Input: part model. Units: mm. Frame: model coordinates. A direction names the side the tool comes from. Round coordinates to 2 decimals unless told otherwise and drop trailing zeros. Loops run counter-clockwise (first coordinate to the right, second up) from the corner with the lowest first, then second, coordinate; pieces in that order, holes last. Notation, with made-up numbers: (-2, 27.5) -> (24, 27.5) arc R28 cw to (24, 65.5) -> close; hole circle Ø10 at (-1, -37.5). An arc over 180 degrees is marked (long way). Answer in a Markdown table with one row per item. Add a question column.
Q1. Pin query (flat end, axial travel): pin 1 (1.8 mm diameter, centred on x = 4.5, y = 4.5, fed in from -Z); pin 2 (2.5 mm diameter, centred on x = 2, z = -58, fed in from -Y); pin 3 (9 mm diameter, centred on y = 15.25, z = -4, fed in from +X). Return the tip coordinate at first contact, or that it passes through.
Q2. Section C-C, the plane y = 21.25. Output: boundary loops of the cut face in (x, z).
Q3. Ray query, L1, parallel to Z at x = 2.4, y = 15.25; L2, parallel to Z at x = 2.3, y = 18.25; L3, parallel to Y at x = 3.8, z = -52. Return the intervals inside material, ascending. Write a range as from..to.
Q4. Reachability of faces 5 (the face through (3, 6.25, 1)), 6 (the face through (3, 6.25, -57)), 7 (the face through (3, 14, -59)), 8 (the face through (3, 22.25, 1)), 9 (the face through (3, 21, -6.25)) from +Z, -Z, +X, -X, +Y, -Y: full face, straight path, thin tool, end or side. Return the list, or none.
Q5. Section D-D, the plane z = -4. Output: boundary loops of the cut face in (x, y).
Q6. Section A-A, the plane y = 15.25. Output: boundary loops of the cut face in (x, z), and give its area (3 significant figures).
Q7. Section B-B, the plane x = 2.8. Output: boundary loops of the cut face in (y, z).
Q8. Mould query, pull axis Z, two halves, no side actions, for faces 1 (the face through (2.958, 10.254, -3.813)), 2 (the face through (3, 3, -56)), 3 (the face through (3, 3, 0)), 4 (the face through (3, 21, -1.75)). Classes: pulls with the +Z half, pulls with the -Z half, needs draft (parallel to the pull), parting line crosses it, or undercut.
```python
from build123d import *

# Parameters (mm, degrees)
SKETCH1_W           = 6
SKETCH1_H           = 56
BOSS_EXTRUDE1_DEPTH = 22.25
SKETCH6_W           = 6
SKETCH6_H           = 16
BOSS_EXTRUDE3_DEPTH = 3
CUT_EXTRUDE1_DEPTH  = 6


with BuildPart() as part:
    # Sketch1 → Boss-Extrude1 (new body)
    with BuildSketch(Plane(origin=(0, 0, 0), x_dir=(1, 0, 0), z_dir=(0, 1, 0))):
        with Locations((3, 28)):
            Rectangle(SKETCH1_W, SKETCH1_H)
    extrude(amount=BOSS_EXTRUDE1_DEPTH)

    # Sketch6 → Boss-Extrude3 (add)
    with BuildSketch(Plane(origin=(0, 0, -56), x_dir=(-1, 0, 0), z_dir=(0, 0, -1))):
        with Locations((-3, 14.25)):
            Rectangle(SKETCH6_W, SKETCH6_H)
    boss_extrude3 = extrude(amount=BOSS_EXTRUDE3_DEPTH)

    # Mirror3: Boss-Extrude3 across plane
    add(boss_extrude3.mirror(Plane(origin=(0, 0, -28), x_dir=(1, 0, 0), z_dir=(0, 0, -1))))

    # Sketch7 → Cut-Extrude1 (cut)
    with BuildSketch(Plane.ZY):
        with BuildLine():
            Line((-54.25, 19.715142775), (-54.25, 24.715142775))
            Line((-54.25, 24.715142775), (-49.75, 24.715142775))
            Line((-49.75, 24.715142775), (-49.75, 19.715142775))
            ThreePointArc((-49.75, 19.715142775), (-52, 10.25), (-54.25, 19.715142775))
        make_face()
        with BuildLine():
            Line((-6.25, 19.715142775), (-6.25, 24.715142775))
            Line((-6.25, 24.715142775), (-1.75, 24.715142775))
            Line((-1.75, 24.715142775), (-1.75, 19.715142775))
            ThreePointArc((-1.75, 19.715142775), (-4, 10.25), (-6.25, 19.715142775))
        make_face()
    extrude(amount=-CUT_EXTRUDE1_DEPTH, mode=Mode.SUBTRACT)


solid = part.part
```
Answer block:
| question | item | result |
|---|---|---|
| 1 | pin 1 | z = -56 |
| 1 | pin 2 | y = 6.25 |
| 1 | pin 3 | through |
| 2 | outline | (0, -59) -> (6, -59) -> (6, -54.25) -> (0, -54.25) -> close; (0, -49.75) -> (6, -49.75) -> (6, -6.25) -> (0, -6.25) -> close; (0, -1.75) -> (6, -1.75) -> (6, 3) -> (0, 3) -> close |
| 3 | L1 | -59..-57, -47..-9, 1..3 |
| 3 | L2 | -59..-56, -48..-8, 0..3 |
| 3 | L3 | 0..10.25 |
| 4 | face 5 | +Z, +X, -X, -Y |
| 4 | face 6 | -Z, +X, -X, -Y |
| 4 | face 7 | -Z, +X, -X, +Y, -Y |
| 4 | face 8 | +Z, -Z, +X, -X, +Y |
| 4 | face 9 | +X, -X, +Y |
| 5 | outline | (0, 0) -> (6, 0) -> (6, 10.25) -> (0, 10.25) -> close |
| 6 | outline | (0, -59) -> (6, -59) -> (6, -57) -> (0, -57) -> close; (0, -47) -> (6, -47) -> (6, -9) -> (0, -9) -> close; (0, 1) -> (6, 1) -> (6, 3) -> (0, 3) -> close |
| 6 | area | 252 mm^2 |
| 7 | outline | (0, -56) -> (6.25, -56) -> (6.25, -59) -> (22.25, -59) -> (22.25, -54.25) -> (19.72, -54.25) arc R5 cw (long way) to (19.72, -49.75) -> (22.25, -49.75) -> (22.25, -6.25) -> (19.72, -6.25) arc R5 cw (long way) to (19.72, -1.75) -> (22.25, -1.75) -> (22.25, 3) -> (6.25, 3) -> (6.25, 0) -> (0, 0) -> close |
| 8 | face 1 | undercut |
| 8 | face 2 | pulls with the -Z half |
| 8 | face 3 | pulls with the +Z half |
| 8 | face 4 | undercut |
